Design review of the part built by this model. Coordinates are the model's own, in mm. A direction names the side the tool comes from. Coordinates: 2 decimals unless noted, no trailing zeros. Write each loop counter-clockwise with the first axis right and the second up, starting at its lowest first coordinate (ties: lowest second). Pieces come first, ordered by that corner, then holes. Notation, with made-up numbers: M -11,-13.5 L 8,-13.5 A15 cw 8,-1.5 Z; hole C 33,4.25 d1. An arc over 180 degrees is marked long. Return JSON: item names as keys, results as strings. Group by question number.
```python
from build123d import *

# Parameters (mm, degrees)
F1_DEPTH = 20
F2_R     = 0.5


with BuildPart() as f1:
    # F0 (on Top) → F1 (new body)
    with BuildSketch(Plane.XY):
        with BuildLine():
            ThreePointArc((9.625, -4.5), (9.107562, -5.472014), (8.492301, -6.385253))
            Line((8.492301, -6.385253), (9.779271, -6.385253))
            Line((9.779271, -6.385253), (10.759093, -4.872048))
            ThreePointArc((10.759093, -4.872048), (10.938513, -4.481831), (11, -4.056767))
            Line((11, -4.056767), (11, 15.625))
            Line((11, 15.625), (-11, 15.625))
            Line((-11, 15.625), (-11, -4.056767))
            ThreePointArc((-11, -4.056767), (-10.938513, -4.481831), (-10.759093, -4.872048))
            Line((-10.759093, -4.872048), (-9.779271, -6.385253))
            Line((-9.779271, -6.385253), (-8.492301, -6.385253))
            ThreePointArc((-8.492301, -6.385253), (-9.107562, -5.472014), (-9.625, -4.5))
            ThreePointArc((-9.625, -4.5), (-10.625, 0), (-9.625, 4.5))
            ThreePointArc((-9.625, 4.5), (0, 10.625), (9.625, 4.5))
            ThreePointArc((9.625, 4.5), (10.625, 0), (9.625, -4.5))
        make_face()
        with BuildLine():
            Line((-9.625, -4.5), (-9.625, 4.5))
            ThreePointArc((-9.625, 4.5), (-10.625, 0), (-9.625, -4.5))
        make_face()
        with BuildLine():
            Line((9.625, 4.5), (9.625, -4.5))
            ThreePointArc((9.625, -4.5), (10.625, 0), (9.625, 4.5))
        make_face()
    extrude(amount=F1_DEPTH)

    # F2
    f2_edges = [f1.edges().sort_by_distance(p)[0] for p in [
        (-9.779271, -6.385253, 10),
        (9.779271, -6.385253, 10),
    ]]
    fillet(f2_edges, radius=F2_R)


solid = f1.part
```
Item 1: Machinability: for faces 1 (the flat face through (11, 6, 10)), 2 (the cylindrical face through (9.115, -5.459, 9.86)), which of the approach directions +Z, -Z, +X, -X, +Y, -Y give a long, thin tool a straight path to every point of the face, cutting with its end or side? Answer none if there is none.
Item 2: Add section B-B (z = 11.5). Write out the cut boundary in (x, y) (3 decimals), plus the area to 3 significant figures.
Item 3: Add section A-A (y = 0). Write out the cut boundary in (x, z) (3 decimals), plus the area to 3 significant figures.
Item 4: Add section C-C (y = 6). Write out the cut boundary in (x, z), plus the area to 3 significant figures.
Item 5: For pin 1 (6 mm diameter, centred on x = 1.5, z = 7.5, fed in from -Y) (3 decimals); pin 2 (3 mm diameter, centred on x = -5, z = 6, fed in from -Y), all flat-tipped, find the tip position at first contact; note any pin that passes through.
Item 6: Add section D-D (x = 4.5). Write out the cut boundary in (y, z) (3 decimals).
Item 7: For line 1 (X direction, y = -3, z = 16.5) (3 decimals); line 2 (X direction, y = 8.75, z = 14.5); line 3 (Y direction, x = -7.5, z = 5.5) (3 decimals), list the stretches that pass through material, from the lowest coordinate up.
Item 8: The part is to be moulded in two halves that separate along Y. For faces 3 (the flat face through (9.625, 0, 10)), 4 (the flat face through (9, -6.385, 10)), 5 (the flat face through (-11, 6, 10)), say which applies: pulls with the +Y half, pulls with the -Y half, needs draft (parallel to the pull), parting line crosses it, or undercut.
Geometry check:
{
 "1": {"face 1": "+Z, -Z, +X, +Y, -Y", "face 2": "+Z, -Z"},
 "2": {"outline": "M -11,-4.057 A1.5 ccw -10.759,-4.872 L -9.927,-6.157 A0.5 ccw -9.507,-6.385 L -8.492,-6.385 A10.625 cw -9.625,-4.5 L -9.625,4.5 A10.625 cw 9.625,4.5 L 9.625,-4.5 A10.625 cw 8.492,-6.385 L 9.507,-6.385 A0.5 ccw 9.927,-6.157 L 10.759,-4.872 A1.5 ccw 11,-4.057 L 11,15.625 L -11,15.625 Z", "area": "190 mm^2"},
 "3": {"outline": "M -11,0 L -9.625,0 L -9.625,20 L -11,20 Z; M 9.625,0 L 11,0 L 11,20 L 9.625,20 Z", "area": "55.0 mm^2"},
 "4": {"outline": "M -11,0 L -8.77,0 L -8.77,20 L -11,20 Z; M 8.77,0 L 11,0 L 11,20 L 8.77,20 Z", "area": "89.3 mm^2"},
 "5": {"pin 1": "y = 9.625", "pin 2": "y = 8.4"},
 "6": {"outline": "M 9.625,0 L 15.625,0 L 15.625,20 L 9.625,20 Z"},
 "7": {"line 1": "-11 to -9.625, 9.625 to 11", "line 2": "-11 to -6.03, 6.03 to 11", "line 3": "7.526 to 15.625"},
 "8": {"face 3": "undercut", "face 4": "pulls with the -Y half", "face 5": "needs draft"}
}
